CAD build for the part. Positions are in the model's coordinates, mm. Face numbers are marked on the shaded views. A direction names the side the tool comes from. Round coordinates to 2 decimals unless told otherwise and drop trailing zeros. Order: outer loops, then holes, each group sorted by start corner. A loop starts at its lowest first (then second) coordinate and runs counter-clockwise, first axis right, second up. Notation, with made-up numbers: (76.25, 52.25) - (99.25, 52.25) arc R16 cw to (99.25, 80.25) - close; hole circle Ø3 at (62.25, 6.5). An arc over 180 degrees is marked (long way). Write item = value, one per line.
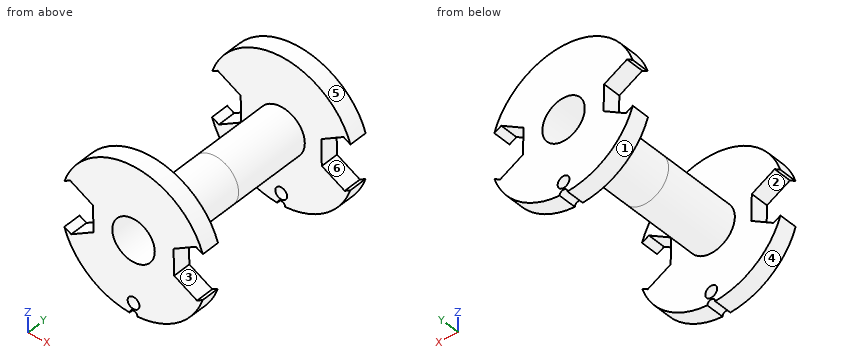
from build123d import *

# Parameters (mm, degrees)
SKETCH1_R           = 9.25
SKETCH1_R_2         = 2.7
BOSS_EXTRUDE1_DEPTH = 2.3
CUT_EXTRUDE3_DEPTH  = 2.5
SKETCH4_R           = 0.75
SKETCH4_R_2         = 0.5
CUT_EXTRUDE4_DEPTH  = 5
SKETCH2_R           = 3
SKETCH2_R_2         = 2.7
BOSS_EXTRUDE2_DEPTH = 10


with BuildPart() as part:
    # Sketch1 → Boss-Extrude1 (new body)
    with BuildSketch(Plane(origin=(0, 0, 0), x_dir=(1, 0, 0), z_dir=(0, 1, 0))):
        Circle(SKETCH1_R)
        Circle(SKETCH1_R_2, mode=Mode.SUBTRACT)
    extrude(amount=BOSS_EXTRUDE1_DEPTH)

    # Sketch3 → Cut-Extrude3 (cut)
    with BuildSketch(Plane.XZ):
        Polygon((-5.161329605, 1.721273866), (-8.071331697, 3.318997608), (-10.910002092, 1.597723742), (-10.838670395, -1.721273866), (-7.928668303, -3.318997608), (-5.089997908, -1.597723742), align=None)
        Polygon((5.161329605, -1.721273866), (8.071331697, -3.318997608), (10.910002092, -1.597723742), (10.838670395, 1.721273866), (7.928668303, 3.318997608), (5.089997908, 1.597723742), align=None)
    extrude(amount=-CUT_EXTRUDE3_DEPTH, mode=Mode.SUBTRACT)

    # Sketch4 → Cut-Extrude4 (cut)
    with BuildSketch(Plane(origin=(0, 2.3, 0), x_dir=(1, 0, 0), z_dir=(0, 1, 0))):
        with Locations((0, 7.8)):
            Circle(SKETCH4_R)
        with Locations((0, 9.25)):
            Circle(SKETCH4_R_2)
    extrude(amount=-CUT_EXTRUDE4_DEPTH, mode=Mode.SUBTRACT)

    # Sketch2 → Boss-Extrude2 (add)
    with BuildSketch(Plane(origin=(0, 2.3, 0), x_dir=(1, 0, 0), z_dir=(0, 1, 0))):
        Circle(SKETCH2_R)
        Circle(SKETCH2_R_2, mode=Mode.SUBTRACT)
    extrude(amount=BOSS_EXTRUDE2_DEPTH)

    # Mirror7: part across plane


with BuildPart() as part_1:
    add(part.part)
    add(part.part.mirror(Plane.ZX.offset(12.3)))


solid = part_1.part
(1) Probe line 1 along Z through (x, y) = (0, 23.55); line 2 along Y through (x, z) = (1.5, 4.5); line 3 along Z through (x, y) = (0, 3.5). List the from-to ranges inside material, lowest first.
Solved:
line_1 = -8.75 to -8.55, -7.05 to -2.7, 2.7 to 9.25
line_2 = 0 to 2.3, 22.3 to 24.6
line_3 = -3 to -2.7, 2.7 to 3
(2) Drop flat-ended pins along their axis: pin 1 (10 mm diameter, centred on x = 3, y = 17.5, fed in from -Z); pin 2 (6 mm diameter, centred on x = 2.5, y = 11.5, fed in from +Z). Give the stop position or say it passes through.
Solved:
pin_1 = -9.11
pin_2 = 3
(3) Band-saw the part on A-A on x = 5.75. List the corners of the cut face in (y, z), plus the area to 3 significant figures.
Solved:
outline = (0, -7.25) - (2.3, -7.25) - (2.3, -2.04) - (0, -2.04) - close; (0, 2) - (2.3, 2) - (2.3, 7.25) - (0, 7.25) - close; (22.3, -7.25) - (24.6, -7.25) - (24.6, -2.04) - (22.3, -2.04) - close; (22.3, 2) - (24.6, 2) - (24.6, 7.25) - (22.3, 7.25) - close
area = 48.1 mm²
(4) Tool access for the marked faces 1 and 2: list every direction of +Z, -Z, +X, -X, +Y, -Y with a clear straight run to the whole face (end or side of a thin tool).
Solved:
face_1 = -Z, -X, +Y, -Y
face_2 = +Y, -Y
(5) Band-saw the part on B-B on z = -6.5. List the corners of the cut face in (x, y).
Solved:
outline = (-6.58, 0) - (6.58, 0) - (6.58, 2.3) - (-6.58, 2.3) - close; (-6.58, 22.3) - (6.58, 22.3) - (6.58, 24.6) - (-6.58, 24.6) - close
(6) Band-saw the part on D-D on y = 4.25. List the corners of the cut face in (x, z), plus the area to 3 significant figures.
Solved:
outline = circle Ø6 at (0, 0); hole circle Ø5.4 at (0, 0)
area = 5.37 mm²
(7) Pull direction X, two halves, no side cores. Call the marked faces 3, 4, 5 and 6: released by +X, released by -X, zero draft, split by the parting line, or undercut.
Solved:
face_3 = undercut
face_4 = released by -X
face_5 = split by the parting line
face_6 = undercut
(8) Band-saw the part on C-C on x = -1.5. List the corners of the cut face in (y, z) (3 decimals).
Solved:
outline = (0, -9.128) - (2.3, -9.128) - (2.3, -2.598) - (22.3, -2.598) - (22.3, -9.128) - (24.6, -9.128) - (24.6, -2.245) - (0, -2.245) - close; (0, 2.245) - (24.6, 2.245) - (24.6, 9.128) - (22.3, 9.128) - (22.3, 2.598) - (2.3, 2.598) - (2.3, 9.128) - (0, 9.128) - close
